Autodesk Inventor part; units mm, degrees
ref_plane "YZ Plane" through (0, 0, 0) normal (1, 0, 0) x (0, 1, 0)
ref_plane "XZ Plane" through (0, 0, 0) normal (0, 1, 0) x (-1, 0, 0)
ref_plane "XY Plane" through (0, 0, 0) normal (0, 0, 1) x (1, 0, 0)
sketch "Sketch1" plane through (0, 0, 0) normal (0, 1, 0) x (-1, 0, 0)
  line L0 (0, 0) -> (16, 0)
  line L1 (16, 0) -> (16, -3.2)
  line L2 (16, -3.2) -> (3.2, -3.2)
  line L3 (0, -3.2) -> (0, 0)
  line L4 (0, 0) -> (3.2, 0)
  line L5 (3.2, -3.2) -> (3.2, -16)
  line L6 (3.2, -16) -> (0, -16)
  line L7 (0, -16) -> (0, 0)
  dimension "d0" = 16
  dimension "d1" = 3.2
  dimension "d2" = 3.2
  dimension "d3" = 16
extrude "Extrusion1" add sketch "Sketch1" along normal blind 40
fillet "Fillet1" radius 2 4 edges at (-1.6, 40, -16) (-16, 40, -1.6) (-1.6, 0, -16) (-16, 0, -1.6)
sketch "Sketch4" plane through (0, 0, 0) normal (1, 0, 0) x (0, 0, -1)
  circle A0 centre (9.6, 16) radius 1.85
  circle A1 centre (9.6, 32) radius 1.85
  point P0 (0, 0)
sketch "Sketch5" plane through (0, 0, 0) normal (0, 0, 1) x (1, 0, 0)
  circle A0 centre (-9.6, 16) radius 1.85
  circle A1 centre (-9.6, 32) radius 1.85
  point P0 (0, 0)
extrude "Extrusion4" cut sketch "Sketch4" against normal through all
extrude "Extrusion5" cut sketch "Sketch5" against normal through all
properties part number "wheelguardbracket"
Work out the finished part from the listing and answer in its coordinate system (mm). A direction names the side the tool comes from. Give positions to 0.01 mm unless a question says otherwise; leave off trailing zeros. Loops run counter-clockwise (first coordinate to the right, second up) from the corner with the lowest first, then second, coordinate; pieces in that order, holes last. Notation, with made-up numbers: (-23, 5) - (27, 5) arc R14 cw to (27, 23) - close; hole circle Ø3 at (-29, 49). An arc over 180 degrees is marked (long way). Answer in a Markdown table with one row per item.
(1) A tool of negligible diameter and unlimited length cuts with its end or side. For faces 1 (the face through (-3.2, 20, -10)), 2 (the face through (-10.964, 33.25, -1.578)), from which of +Z, -Z, +X, -X, +Y, -Y can it reach the whole face along a straight path? Write none if from no direction.
Results list:
| item | result |
|---|---|
| face 1 | -Z, -X, +Y, -Y |
| face 2 | +Z, -Z |
(2) Section B-B (x = -9.6) is taken. Give the vertices of the cut face in (y, z).
Results list:
| item | result |
|---|---|
| outline | (0, -3.2) - (14.15, -3.2) - (14.15, 0) - (0, 0) - close; (17.85, -3.2) - (30.15, -3.2) - (30.15, 0) - (17.85, 0) - close; (33.85, -3.2) - (40, -3.2) - (40, 0) - (33.85, 0) - close |
(3) For a pull along Y with two mould halves and no side action, classify faces 3 (the face through (-1.58, 0.57, -15.4)), 4 (the face through (-10.964, 17.25, -1.578)), 5 (the face through (-15.43, 39.4, -1.62)) as pulls with the +Y half, pulls with the -Y half, needs draft (parallel to the pull), parting line crosses it, or undercut.
Results list:
| item | result |
|---|---|
| face 3 | pulls with the -Y half |
| face 4 | undercut |
| face 5 | pulls with the +Y half |
(4) Section C-C (z = -8.25) is taken. Give the vertices of the cut face in (x, y).
Results list:
| item | result |
|---|---|
| outline | (-3.2, 0) - (0, 0) - (0, 14.74) - (-3.2, 14.74) - close; (-3.2, 17.26) - (0, 17.26) - (0, 30.74) - (-3.2, 30.74) - close; (-3.2, 33.26) - (0, 33.26) - (0, 40) - (-3.2, 40) - close |
(5) Section A-A (y = 32) is taken. Give the vertices of the cut face in (x, z), and give its area (3 significant figures).
Results list:
| item | result |
|---|---|
| outline | (-16, -3.2) - (-11.45, -3.2) - (-11.45, 0) - (-16, 0) - close; (-7.75, -3.2) - (-3.2, -3.2) - (-3.2, -7.75) - (0, -7.75) - (0, 0) - (-7.75, 0) - close; (-3.2, -16) - (0, -16) - (0, -11.45) - (-3.2, -11.45) - close |
| area | 68.5 mm² |
(6) Consider L1, parallel to Y at x = -2.2, z = -9.6; L2, parallel to X at y = 31.5, z = -3.5. Determine where each line is inside the solid, lowest interval first. Write a range as [from, to].
Results list:
| item | result |
|---|---|
| L1 | y = [0, 14.15], [17.85, 30.15], [33.85, 40] |
| L2 | x = [-3.2, 0] |
(7) Section D-D (x = -12.5) is taken. Give the vertices of the cut face in (y, z), and give its area (3 significant figures).
Results list:
| item | result |
|---|---|
| outline | (0, -3.2) - (40, -3.2) - (40, 0) - (0, 0) - close |
| area | 128 mm² |
(8) Flat-ended cylindrical pins translate along their axes: pin 1 Ø1.5 at (x, z) = (-7.5, -5.5) entering from +Y; pin 2 Ø5 at (y, z) = (32, -9.6) entering from -X; pin 3 Ø5 at (x, y) = (-9.6, 32) entering from -Z. Find the tip coordinate at first contact, or state that the pin passes through.
Results list:
| item | result |
|---|---|
| pin 1 | passes through |
| pin 2 | stops at x = -3.2 |
| pin 3 | stops at z = -3.2 |
